Source: CAD feature listing. Evaluate the final solid. Frame: model axes, mm. A direction names the side the tool comes from. Give positions to 0.01 mm unless a question says otherwise; leave off trailing zeros. Loops run counter-clockwise (first coordinate to the right, second up) from the corner with the lowest first, then second, coordinate; pieces in that order, holes last. Notation, with made-up numbers: (-10.75, -5.5) - (-0.75, -5.5) arc R10 cw to (-0.75, 2.5) - close; hole circle Ø11 at (11, -39). An arc over 180 degrees is marked (long way). Write each question's results on one line, items separated by ' | '. Start each with the question number.
(1) Reachability of faces 4 (the cylindrical face through (92.5, 41.1, 30.32)), 5 (the flat face through (47, 42, 25.75)) from +Z, -Z, +X, -X, +Y, -Y: full face, straight path, thin tool, end or side. Return the list, or none.
(2) Material intervals for line 1 along X through (y, z) = (12, -8); line 2 along X through (y, z) = (63, 25); line 3 along X through (y, z) = (58.65, 0), sorted ascending. Write a range as [from, to].
(3) Cut plane D-D on x = 99. Return the cut outline in (y, z) (3 decimals).
(4) Pull-direction query (X, two-part tool) for faces 1 (the cylindrical face through (47.59, 1.5, 30.32)), 2 (the cylindrical face through (87.656, 70.75, -25.227)), 3 (the flat face through (104, 25, -4)); classes: pulls with the +X half, pulls with the -X half, needs draft (parallel to the pull), parting line crosses it, or undercut.
(5) Cut plane A-A on y = 12. Give the number of separate pieces and of enclosed holes in the cut face, then the cut area to 3 significant figures.
(6) Contact query for flat-ended pins moving along their axis: pin 1 (5 mm diameter, centred on x = 57, z = 22, fed in from +Y); pin 2 (15.5 mm diameter, centred on x = 67, z = 6, fed in from +Y); pin 3 (10.5 mm diameter, centred on y = 50.5, z = -0.5, fed in from +X); pin 4 (6.5 mm diameter, centred on x = 85.5, z = 23.25, fed in from +Y). Output: stop coordinate, or through.
(7) Cut plane B-B on x = 20.5. Return the cut outline in (y, z), then the cut area to 3 significant figures.
(8) Cut plane C-C on x = 69. Return the cut outline in (y, z), then the cut area to 3 significant figures.
from build123d import *

# Parameters (mm, degrees)
SKETCH1_W                 = 94
SKETCH1_H                 = 63.5
BOSS_EXTRUDE1_DEPTH       = 76.2
SKETCH2_W                 = 82.000024
SKETCH2_H                 = 51.500024
CUT_EXTRUDE1_DEPTH        = 70.2
SKETCH7_R                 = 33
CUT_EXTRUDE4_DEPTH        = 4
SKETCH8_R                 = 12.55
CUT_EXTRUDE5_DEPTH        = 2
SKETCH15_W                = 72
SKETCH15_H                = 25
BOSS_EXTRUDE3_DEPTH       = 22
FILLET1_R                 = 5
BOSS_EXTRUDE4_DEPTH       = 70.2
F_1_0MM_DOWEL_HOLE2_D     = 5.85
F_1_0MM_DOWEL_HOLE2_DEPTH = 10.75
F_1_0MM_DOWEL_HOLE2_TIP   = 1.757517311
SKETCH49_R                = 15.875
CUT_EXTRUDE7_DEPTH        = 5.999988
BOSS_EXTRUDE5_START       = 10
SKETCH51_R                = 18.875
SKETCH51_R_2              = 15.875
BOSS_EXTRUDE5_DEPTH       = 10
SKETCH52_R                = 2.75
CUT_EXTRUDE8_DEPTH        = 124.940865436
SKETCH53_R                = 23.17
CUT_EXTRUDE9_DEPTH        = 1.999988
BRACKET_HOLES_D           = 4
BRACKET_HOLES_DEPTH       = 10.75
BRACKET_HOLES_TIP         = 1.201721238


with BuildPart() as part:
    # Sketch1 → Boss-Extrude1 (new body)
    with BuildSketch(Plane(origin=(0, 0, 0), x_dir=(1, 0, 0), z_dir=(0, 1, 0))):
        with Locations((47, 0)):
            Rectangle(SKETCH1_W, SKETCH1_H)
    extrude(amount=BOSS_EXTRUDE1_DEPTH)

    # Sketch2 → Cut-Extrude1 (cut)
    with BuildSketch(Plane(origin=(0, 76.2, 0), x_dir=(1, 0, 0), z_dir=(0, 1, 0))):
        with Locations((47, 0)):
            Rectangle(SKETCH2_W, SKETCH2_H)
    extrude(amount=-CUT_EXTRUDE1_DEPTH, mode=Mode.SUBTRACT)

    # Sketch7 → Cut-Extrude4 (cut)
    with BuildSketch(Plane(origin=(0, 0, -31.75), x_dir=(-1, 0, 0), z_dir=(0, 0, -1))):
        with Locations((-38.1, 38.1)):
            Circle(SKETCH7_R)
    extrude(amount=-CUT_EXTRUDE4_DEPTH, mode=Mode.SUBTRACT)

    # Sketch8 → Cut-Extrude5 (cut)
    with BuildSketch(Plane.XY.offset(-25.750012)):
        with Locations((38.1, 38.1)):
            Circle(SKETCH8_R)
    extrude(amount=-CUT_EXTRUDE5_DEPTH, mode=Mode.SUBTRACT)

    # Sketch15 → Boss-Extrude3 (add)
    with BuildSketch(Plane(origin=(0, 28, 0), x_dir=(1, 0, 0), z_dir=(0, 1, 0))):
        with Locations((48.25, -3.399988)):
            Rectangle(SKETCH15_W, SKETCH15_H)
    extrude(amount=-BOSS_EXTRUDE3_DEPTH)

    # Fillet1
    fillet1_edges = [part.edges().sort_by_distance(p)[0] for p in [
        (47, 0, -31.75),
        (94, 0, 0),
        (47, 0, 31.75),
        (0, 0, 0),
        (0, 38.1, -31.75),
        (94, 38.1, -31.75),
        (94, 38.1, 31.75),
        (0, 38.1, 31.75),
    ]]
    fillet(fillet1_edges, radius=FILLET1_R)

    # Sketch44 → Boss-Extrude4 (add)
    with BuildSketch(Plane(origin=(0, 76.2, 0), x_dir=(1, 0, 0), z_dir=(0, 1, 0))):
        with BuildLine():
            Line((8.499988, 17.250012), (5.999988, 17.250012))
            Line((5.999988, 17.250012), (5.999988, 25.750012))
            Line((5.999988, 25.750012), (14.499988, 25.750012))
            Line((14.499988, 25.750012), (14.499988, 23.250012))
            ThreePointArc((14.499988, 23.250012), (12.742628687, 19.007371313), (8.499988, 17.250012))
        make_face()
        with BuildLine():
            Line((8.499988, -17.250012), (5.999988, -17.250012))
            Line((5.999988, -17.250012), (5.999988, -25.750012))
            Line((5.999988, -25.750012), (14.499988, -25.750012))
            Line((14.499988, -25.750012), (14.499988, -23.250012))
            ThreePointArc((14.499988, -23.250012), (12.742628687, -19.007371313), (8.499988, -17.250012))
        make_face()
        with BuildLine():
            Line((79.500012, -23.250012), (79.500012, -25.750012))
            Line((79.500012, -25.750012), (88.000012, -25.750012))
            Line((88.000012, -25.750012), (88.000012, -17.250012))
            Line((88.000012, -17.250012), (85.500012, -17.250012))
            ThreePointArc((85.500012, -17.250012), (81.257371313, -19.007371313), (79.500012, -23.250012))
        make_face()
        with BuildLine():
            Line((79.500012, 23.250012), (79.500012, 25.750012))
            Line((79.500012, 25.750012), (88.000012, 25.750012))
            Line((88.000012, 25.750012), (88.000012, 17.250012))
            Line((88.000012, 17.250012), (85.500012, 17.250012))
            ThreePointArc((85.500012, 17.250012), (81.257371313, 19.007371313), (79.500012, 23.250012))
        make_face()
    extrude(amount=-BOSS_EXTRUDE4_DEPTH)

    # Ø1.0mm Dowel Hole2
    with Locations(Plane(origin=(0, 76.2, 0), x_dir=(1, 0, 0), z_dir=(0, 1, 0))):
        with Locations((8.499988, 23.250012), (8.499988, -23.250012), (85.500012, -23.250012), (85.500012, 23.250012)):
            Hole(F_1_0MM_DOWEL_HOLE2_D / 2, depth=F_1_0MM_DOWEL_HOLE2_DEPTH)
            with Locations((0, 0, -(F_1_0MM_DOWEL_HOLE2_DEPTH + F_1_0MM_DOWEL_HOLE2_TIP / 2))):  # 118° drill point
                Cone(0, F_1_0MM_DOWEL_HOLE2_D / 2, F_1_0MM_DOWEL_HOLE2_TIP, mode=Mode.SUBTRACT)

    # Sketch49 → Cut-Extrude7 (cut)
    with BuildSketch(Plane(origin=(94, 0, 0), x_dir=(0, 0, -1), z_dir=(1, 0, 0))):
        with Locations((0, 40.6)):
            Circle(SKETCH49_R)
    extrude(amount=-CUT_EXTRUDE7_DEPTH, mode=Mode.SUBTRACT)

    # Sketch51 → Boss-Extrude5 (add)
    with BuildSketch(Plane(origin=(94, 0, 0), x_dir=(0, 0, -1), z_dir=(1, 0, 0)).offset(BOSS_EXTRUDE5_START)):
        with Locations(Location((0, 40.6, 0), (0, 0, 180))):
            Circle(SKETCH51_R)
        with Locations((0, 40.6)):
            Circle(SKETCH51_R_2, mode=Mode.SUBTRACT)
    extrude(amount=-BOSS_EXTRUDE5_DEPTH)

    # Sketch52 → Cut-Extrude8 (cut, through all)
    with BuildSketch(Plane(origin=(0, 59.475, 0), x_dir=(-1, 0, 0), z_dir=(0, 1, 0))):
        with Locations(Location((-99, 0, 0), (0, 0, 90))):
            Circle(SKETCH52_R)
    extrude(amount=-CUT_EXTRUDE8_DEPTH, mode=Mode.SUBTRACT)

    # Sketch53 → Cut-Extrude9 (cut)
    with BuildSketch(Plane(origin=(0, 0, -27.75), x_dir=(-1, 0, 0), z_dir=(0, 0, -1))):
        with Locations((-38.1, 38.1)):
            Circle(SKETCH53_R)
    extrude(amount=-CUT_EXTRUDE9_DEPTH, mode=Mode.SUBTRACT)

    # Bracket Holes
    with Locations(Plane(origin=(0, 28, 0), x_dir=(1, 0, 0), z_dir=(0, 1, 0))):
        with Locations((15.75, 5.100012), (15.75, -2.899988), (80.75, -2.899988), (80.75, 5.100012)):
            Hole(BRACKET_HOLES_D / 2, depth=BRACKET_HOLES_DEPTH)
            with Locations((0, 0, -(BRACKET_HOLES_DEPTH + BRACKET_HOLES_TIP / 2))):  # 118° drill point
                Cone(0, BRACKET_HOLES_D / 2, BRACKET_HOLES_TIP, mode=Mode.SUBTRACT)


solid = part.part
Ans:
1) face 4: +Z, +X, +Y, -Y | face 5: +Y
2) line 1: [0, 6], [12.25, 84.25], [88, 94] | line 2: [0, 14.5], [79.5, 94] | line 3: [0, 6], [88, 96.25], [101.75, 104]
3) outline: (21.926, -2.75) arc R18.875 ccw to (59.274, -2.75) - (56.235, -2.75) arc R15.875 cw to (24.965, -2.75) - close; (21.926, 2.75) - (24.965, 2.75) arc R15.875 cw to (56.235, 2.75) - (59.274, 2.75) arc R18.875 ccw to start
4) face 1: needs draft | face 2: undercut | face 3: pulls with the +X half
5) separate pieces: 2 | enclosed holes: 1 | area: 3,620 mm^2
6) pin 1: y = 6 | pin 2: y = 28 | pin 3: x = 6 | pin 4: y = 76.2
7) outline: (0, -26.75) arc R5 ccw to (5, -31.75) - (10.19, -31.75) - (10.19, -27.75) - (23.03, -27.75) - (23.03, -25.75) - (6, -25.75) - (6, -9.1) - (28, -9.1) - (28, 15.9) - (6, 15.9) - (6, 25.75) - (76.2, 25.75) - (76.2, 31.75) - (5, 31.75) arc R5 ccw to (0, 26.75) - close; (53.17, -27.75) - (66.01, -27.75) - (66.01, -31.75) - (76.2, -31.75) - (76.2, -25.75) - (53.17, -25.75) - close | area: 1,480 mm^2
8) outline: (0, -26.75) arc R5 ccw to (5, -31.75) - (26.52, -31.75) - (26.52, -27.75) - (49.68, -27.75) - (49.68, -31.75) - (76.2, -31.75) - (76.2, -25.75) - (6, -25.75) - (6, -9.1) - (28, -9.1) - (28, 15.9) - (6, 15.9) - (6, 25.75) - (76.2, 25.75) - (76.2, 31.75) - (5, 31.75) arc R5 ccw to (0, 26.75) - close | area: 1,670 mm^2
